from build123d import *

# Parameters (mm, degrees)
F0_R     = 12.25
F1_DEPTH = 6.77
F2_D     = 5.5
F3_D     = 5.3


with BuildPart() as f1:
    # F0 (on Top) → F1 (new body)
    with BuildSketch(Plane.XY):
        Circle(F0_R)
    extrude(amount=-F1_DEPTH)

    # F2 (through all)
    with Locations(Plane.XY):
        with Locations((0, 8.5), (-8.5, 0), (0, -8.5), (8.5, 0)):
            Hole(F2_D / 2)

    # F3 (through all)
    with Locations(Plane.XY):
        with Locations((0, 0)):
            Hole(F3_D / 2)


solid = f1.part
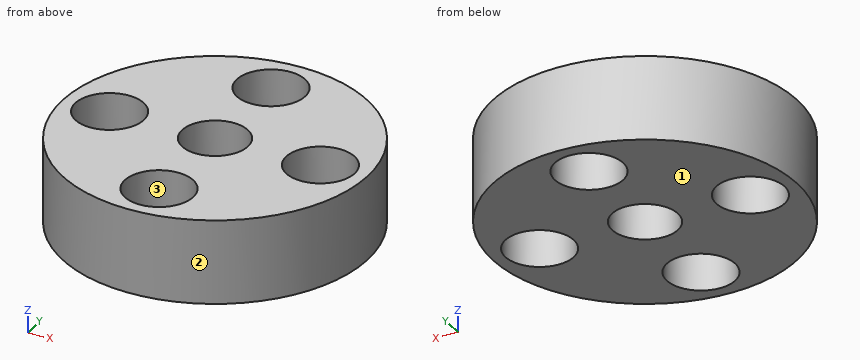
Can you work these out from the model? Positions are in its coordinate system, mm. Face numbers are marked on the shaded views. Give positions to 0.01 mm unless a question says otherwise; leave off trailing zeros. Order: outer loops, then holes, each group sorted by start corner. A loop starts at its lowest first (then second) coordinate and runs counter-clockwise, first axis right, second up. Notation, with made-up numbers: M 27.25,-23.75 L 72.25,-23.75 A30 cw 72.25,2.25 Z; hole C 74,1 d9. An arc over 180 degrees is marked long. Use one line per item in the form item = value. Start each with the question number.
Item 1: If we section it at B-B (y = 7.25): Write out the boundary of the cut face in (x, z).
Item 2: We'd pull the mould along X, two halves only. Please class the marked faces 1, 2 and 3: +X half, -X half, draft (parallel to the pull), parting line (faces both ways), or undercut.
Item 3: Will these pins go through, and if not, where does the flat tip stop? pin 1 Ø1.5 at (x, z) = (4, -5.5) entering from -Y; pin 2 Ø4 at (y, z) = (-9, -2) entering from -X; pin 3 Ø3.5 at (x, y) = (0, -8.5) entering from +Z; pin 4 Ø4 at (x, z) = (-5.5, -3.5) entering from +Y.
Item 4: If we section it at C-C (x = -9.25): Write out the boundary of the cut face in (y, z), then the cut area to 3 significant figures.
Item 5: If I drill on line 1 along Y through (x, z) = (0, -4); line 2 along Y through (x, z) = (1.75, -5); line 3 along X through (y, z) = (-9, -2), over which ranges is the centre line in solid material (lowest first)?
Item 6: If we section it at A-A (x = 0): Write out the boundary of the cut face in (y, z), then the cut area to 3 significant figures.
Item 7: If we section it at D-D (z = -2.25): Write out the boundary of the cut face in (x, y), then the cut area to 3 significant figures.
Outcome:
q1.outline = M -9.87,-6.77 L -2.45,-6.77 L -2.45,0 L -9.87,0 Z; M 2.45,-6.77 L 9.87,-6.77 L 9.87,0 L 2.45,0 Z
q2.face_1 = draft
q2.face_2 = parting line
q2.face_3 = undercut
q3.pin_1 = -11.81
q3.pin_2 = -10.05
q3.pin_3 = through
q3.pin_4 = 11.74
q4.outline = M -8.03,-6.77 L -2.65,-6.77 L -2.65,0 L -8.03,0 Z; M 2.65,-6.77 L 8.03,-6.77 L 8.03,0 L 2.65,0 Z
q4.area = 72.9 mm2
q5.line_1 = -12.25 to -11.25, -5.75 to -2.65, 2.65 to 5.75, 11.25 to 12.25
q5.line_2 = -12.12 to -10.62, -6.38 to -1.99, 1.99 to 6.38, 10.62 to 12.12
q5.line_3 = -8.31 to -2.7, 2.7 to 8.31
q6.outline = M -12.25,-6.77 L -11.25,-6.77 L -11.25,0 L -12.25,0 Z; M -5.75,-6.77 L -2.65,-6.77 L -2.65,0 L -5.75,0 Z; M 2.65,-6.77 L 5.75,-6.77 L 5.75,0 L 2.65,0 Z; M 11.25,-6.77 L 12.25,-6.77 L 12.25,0 L 11.25,0 Z
q6.area = 55.5 mm2
q7.outline = C 0,0 d24.5; hole C -8.5,0 d5.5; hole C 0,-8.5 d5.5; hole C 0,8.5 d5.5; hole C 0,0 d5.3; hole C 8.5,0 d5.5
q7.area = 354 mm2
